Verification items for the finished model (mm, model axes). Face numbers are marked on the shaded views. A direction names the side the tool comes from. Round coordinates to 2 decimals unless told otherwise and drop trailing zeros. Order: outer loops, then holes, each group sorted by start corner. A loop starts at its lowest first (then second) coordinate and runs counter-clockwise, first axis right, second up. Notation, with made-up numbers: (72, -23) -> (100, -23) arc R19 ccw to (100, -9) -> close; hole circle Ø1 at (51, 69). An arc over 180 degrees is marked (long way). Return JSON: item names as keys, results as strings. Group by question number.
1) Section check A-A on z = 11. Enter the section's corners in (x, y), plus the area to 3 significant figures.
2) Scan lines: L1, parallel to Y at x = 3.1, z = 25; L2, parallel to Y at x = 9.5, z = 23; L3, parallel to X at y = 26, z = 11. Record each from-to range of solid material in increasing order.
3) Depth check by flat-ended pin: pin 1 (4 mm diameter, centred on y = 48, z = 34, fed in from -X); pin 2 (0.9 mm diameter, centred on x = 1.5, z = 29, fed in from -Y); pin 3 (2.5 mm diameter, centred on x = 28.7, z = 35, fed in from -Y); pin 4 (1.5 mm diameter, centred on x = 6, y = 47, fed in from +Z). Enter the tip coordinate at first touch or a pass-through.
4) Tool access check on the marked faces 1 and 2. Record the directions out of +Z, -Z, +X, -X, +Y, -Y that give a thin tool (end or side, any length) a straight path to the whole face; none if there is none.
5) Section check B-B on y = 48. Enter the section's corners in (x, z).
6) Draft check along Z on the marked faces 3, 4 and 5. Enter one of: pulls with the +Z half, pulls with the -Z half, needs draft (parallel to the pull), parting line crosses it, or undercut.
7) Section check D-D on y = 7.5. Enter the section's corners in (x, z).
8) Section check C-C on x = 17. Enter the section's corners in (y, z) (3 decimals), plus the area to 3 significant figures.
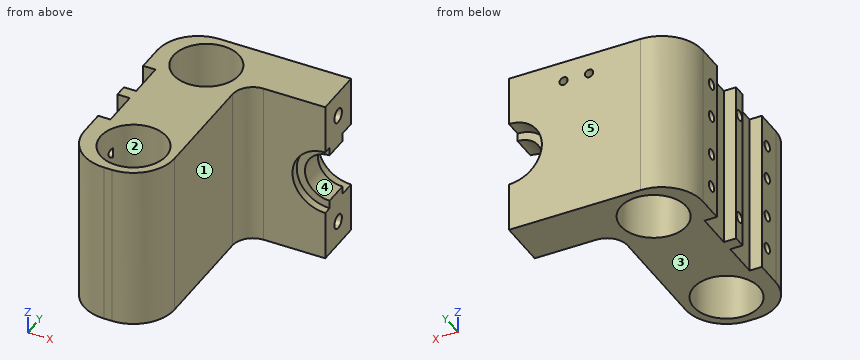
```python
from build123d import *

# Parameters (mm, degrees)
SKETCH1_W           = 22
SKETCH1_H           = 54
SKETCH1_R           = 8
BOSS_EXTRUDE1_DEPTH = 40
SKETCH2_W           = 48
SKETCH2_H           = 21
CUT_EXTRUDE1_DEPTH  = 3
SKETCH6_W           = 40
SKETCH6_H           = 12
BOSS_EXTRUDE2_DEPTH = 20
SKETCH7_R           = 8
CUT_EXTRUDE5_DEPTH  = 4
CUT_EXTRUDE6_START  = -10
SKETCH7_2_R         = 8
CUT_EXTRUDE6_DEPTH  = 3
SKETCH8_R           = 6
CUT_EXTRUDE7_DEPTH  = 7
SKETCH9_R           = 1.75
CUT_EXTRUDE8_DEPTH  = 15
SKETCH10_R          = 1.25
CUT_EXTRUDE9_DEPTH  = 5
SKETCH13_R          = 1.25
CUT_EXTRUDE10_DEPTH = 10
BOSS_EXTRUDE3_START = 3
SKETCH14_W          = 40
SKETCH14_H          = 3
SKETCH14_R          = 1.25
BOSS_EXTRUDE3_DEPTH = 3
FILLET1_R           = 10
FILLET2_R           = 5
SKETCH15_R          = 1
CUT_EXTRUDE11_DEPTH = 10


with BuildPart() as part:
    # Sketch1 → Boss-Extrude1 (new body)
    with BuildSketch(Plane.XY):
        with Locations((11, 27)):
            Rectangle(SKETCH1_W, SKETCH1_H)
        with Locations((12, 10)):
            Circle(SKETCH1_R, mode=Mode.SUBTRACT)
        with Locations((12, 44)):
            Circle(SKETCH1_R, mode=Mode.SUBTRACT)
    extrude(amount=BOSS_EXTRUDE1_DEPTH)

    # Sketch2 → Cut-Extrude1 (cut)
    with BuildSketch(Plane.ZY):
        with Locations((24, 27)):
            Rectangle(SKETCH2_W, SKETCH2_H)
    extrude(amount=-CUT_EXTRUDE1_DEPTH, mode=Mode.SUBTRACT)

    # Sketch6 → Boss-Extrude2 (add)
    with BuildSketch(Plane(origin=(22, 0, 0), x_dir=(0, 0, -1), z_dir=(1, 0, 0))):
        with Locations((-20, 48)):
            Rectangle(SKETCH6_W, SKETCH6_H)
    extrude(amount=BOSS_EXTRUDE2_DEPTH)

    # Sketch7 → Cut-Extrude5 (cut)
    with BuildSketch(Plane(origin=(0, 54, 0), x_dir=(1, 0, 0), z_dir=(0, 1, 0))):
        with Locations((42, -20)):
            Circle(SKETCH7_R)
    extrude(amount=-CUT_EXTRUDE5_DEPTH, mode=Mode.SUBTRACT)

    # Sketch7<2> → Cut-Extrude6 (cut)
    with BuildSketch(Plane(origin=(0, 54, 0), x_dir=(1, 0, 0), z_dir=(0, 1, 0)).offset(CUT_EXTRUDE6_START)):
        with Locations((42, -20)):
            Circle(SKETCH7_2_R)
    extrude(amount=-CUT_EXTRUDE6_DEPTH, mode=Mode.SUBTRACT)

    # Sketch8 → Cut-Extrude7 (cut)
    with BuildSketch(Plane(origin=(0, 50, 0), x_dir=(1, 0, 0), z_dir=(0, 1, 0))):
        with Locations((42, -20)):
            Circle(SKETCH8_R)
    extrude(amount=-CUT_EXTRUDE7_DEPTH, mode=Mode.SUBTRACT)

    # Sketch9 → Cut-Extrude8 (cut)
    with BuildSketch(Plane(origin=(42, 0, 0), x_dir=(0, 0, -1), z_dir=(1, 0, 0))):
        with Locations((-34, 48)):
            Circle(SKETCH9_R)
        with Locations((-6, 48)):
            Circle(SKETCH9_R)
    extrude(amount=-CUT_EXTRUDE8_DEPTH, mode=Mode.SUBTRACT)

    # Sketch10 → Cut-Extrude9 (cut)
    with BuildSketch(Plane.ZY):
        with Locations((33.5, 40)):
            Circle(SKETCH10_R)
        with Locations((33.5, 14)):
            Circle(SKETCH10_R)
        with Locations((6.5, 14)):
            Circle(SKETCH10_R)
        with Locations((6.5, 40)):
            Circle(SKETCH10_R)
        with Locations((15, 40)):
            Circle(SKETCH10_R)
        with Locations((25, 40)):
            Circle(SKETCH10_R)
        with Locations((15, 14)):
            Circle(SKETCH10_R)
        with Locations((25, 14)):
            Circle(SKETCH10_R)
    extrude(amount=-CUT_EXTRUDE9_DEPTH, mode=Mode.SUBTRACT)

    # Sketch13 → Cut-Extrude10 (cut)
    with BuildSketch(Plane.ZY):
        with Locations((6.5, 27)):
            Circle(SKETCH13_R)
        with Locations((33.5, 27)):
            Circle(SKETCH13_R)
    extrude(amount=-CUT_EXTRUDE10_DEPTH, mode=Mode.SUBTRACT)

    # Sketch14 → Boss-Extrude3 (add)
    with BuildSketch(Plane.ZY.offset(-3).offset(BOSS_EXTRUDE3_START)):
        with Locations((20, 27)):
            Rectangle(SKETCH14_W, SKETCH14_H)
        with Locations((6.5, 27)):
            Circle(SKETCH14_R, mode=Mode.SUBTRACT)
        with Locations((33.5, 27)):
            Circle(SKETCH14_R, mode=Mode.SUBTRACT)
    extrude(amount=-BOSS_EXTRUDE3_DEPTH)

    # Fillet1
    fillet1_edges = [part.edges().sort_by_distance(p)[0] for p in [
        (0, 54, 20),
        (22, 0, 20),
        (0, 0, 20),
    ]]
    fillet(fillet1_edges, radius=FILLET1_R)

    # Fillet2
    fillet2_edges = [part.edges().sort_by_distance(p)[0] for p in [
        (22, 42, 20),
    ]]
    fillet(fillet2_edges, radius=FILLET2_R)

    # Sketch15 → Cut-Extrude11 (cut)
    with BuildSketch(Plane(origin=(0, 54, 0), x_dir=(1, 0, 0), z_dir=(0, 1, 0))):
        with Locations(Location((22.5, -35, 0), (0, 0, 180))):
            Circle(SKETCH15_R)
        with Locations(Location((28.7, -35, 0), (0, 0, 180))):
            Circle(SKETCH15_R)
    extrude(amount=-CUT_EXTRUDE11_DEPTH, mode=Mode.SUBTRACT)


solid = part.part
```
Check result:
{
 "1": {"outline": "(0, 10) arc R10 ccw to (10, 0) -> (12, 0) arc R10 ccw to (22, 10) -> (22, 37) arc R5 cw to (27, 42) -> (42, 42) -> (42, 54) -> (10, 54) arc R10 ccw to (0, 44) -> (0, 37.5) -> (3, 37.5) -> (3, 28.5) -> (0, 28.5) -> (0, 25.5) -> (3, 25.5) -> (3, 16.5) -> (0, 16.5) -> close; hole circle Ø16 at (12, 10); hole circle Ø16 at (12, 44)", "area": "913 mm^2"},
 "2": {"L1": "2.76 to 12.75, 15.25 to 38.75, 41.25 to 51.24", "L2": "0.01 to 2.4, 17.6 to 36.4, 51.6 to 53.99", "L3": "0 to 22"},
 "3": {"pin 1": "x = 0.2", "pin 2": "y = 4.07", "pin 3": "y = 42", "pin 4": "through"},
 "4": {"face 1": "+Z, -Z, +X, -Y", "face 2": "+Z, -Z"},
 "5": {"outline": "(0.83, 0) -> (5.07, 0) -> (5.07, 40) -> (0.83, 40) -> close; (18.93, 0) -> (42, 0) -> (42, 4.25) -> (27, 4.25) -> (27, 7.75) -> (42, 7.75) -> (42, 14) arc R6 cw to (42, 26) -> (42, 32.25) -> (27, 32.25) -> (27, 35.75) -> (28.04, 35.75) arc R1 cw to (29.36, 35.75) -> (42, 35.75) -> (42, 40) -> (18.93, 40) -> close; hole circle Ø2 at (22.5, 35)"},
 "6": {"face 3": "pulls with the -Z half", "face 4": "undercut", "face 5": "needs draft"},
 "7": {"outline": "(0.32, 0) -> (4.4, 0) -> (4.4, 40) -> (0.32, 40) -> close; (19.6, 0) -> (21.68, 0) -> (21.68, 40) -> (19.6, 40) -> close"},
 "8": {"outline": "(1.34, 0) -> (3.755, 0) -> (3.755, 40) -> (1.34, 40) -> close; (16.245, 0) -> (37.755, 0) -> (37.755, 40) -> (16.245, 40) -> close; (50.245, 0) -> (54, 0) -> (54, 40) -> (50.245, 40) -> close", "area": "1,110 mm^2"}
}
